from build123d import *

# Parameters (mm, degrees)
SKETCH1_W           = 21.8
SKETCH1_H           = 17.2
BOSS_EXTRUDE1_DEPTH = 1.6
SKETCH2_R           = 0.835
SKETCH2_R_2         = 1.8
CUT_EXTRUDE1_DEPTH  = 1.6


with BuildPart() as part:
    # Sketch1 → Boss-Extrude1 (new body)
    with BuildSketch(Plane.XY):
        Rectangle(SKETCH1_W, SKETCH1_H)
    extrude(amount=BOSS_EXTRUDE1_DEPTH)

    # Sketch2 → Cut-Extrude1 (cut)
    with BuildSketch(Plane.XY.offset(1.6)):
        with Locations((8.89, -7.2)):
            Circle(SKETCH2_R)
        with Locations((6.35, -7.2)):
            Circle(SKETCH2_R)
        with Locations((3.81, -7.2)):
            Circle(SKETCH2_R)
        with Locations((1.27, -7.2)):
            Circle(SKETCH2_R)
        with Locations((-1.27, -7.2)):
            Circle(SKETCH2_R)
        with Locations((-3.81, -7.2)):
            Circle(SKETCH2_R)
        with Locations((-6.35, -7.2)):
            Circle(SKETCH2_R)
        with Locations((-8.89, -7.2)):
            Circle(SKETCH2_R)
        with Locations((-8.3, 6)):
            Circle(SKETCH2_R_2)
    extrude(amount=-CUT_EXTRUDE1_DEPTH, mode=Mode.SUBTRACT)


solid = part.part
Can you work these out from the model? Positions are in its coordinate system, mm. Give positions to 0.01 mm unless a question says otherwise; leave off trailing zeros. Write each loop counter-clockwise with the first axis right and the second up, starting at its lowest first coordinate (ties: lowest second). Pieces come first, ordered by that corner, then holes. Notation, with made-up numbers: M 48.25,13 L 70.25,13 A12 ccw 70.25,33 Z; hole C -17.75,-16 d7. An arc over 180 degrees is marked long. Answer in a Markdown table with one row per item. Add a question column.
Item 1: Please list where these lines run through material, in increasing order: L1, parallel to Y at x = -8.5, z = 1.15; L2, parallel to Y at x = -8.3, z = 0.85; L3, parallel to Y at x = -1.27, z = 1 (3 decimals).
Item 2: Imagine slicing it at D-D, the plane x = -8.89. Write out the boundary of the cut face in (y, z) (3 decimals).
Item 3: Imagine slicing it at B-B, the plane y = 6. Write out the boundary of the cut face in (x, z).
Item 4: Imagine slicing it at C-C, the plane z = 0.3. State how many separate pieces and enclosed holes the cut face has, plus the area to 3 significant figures.
Item 5: For pin 1 Ø1 at (x, y) = (-8.89, -7.2) entering from +Z, with a flat end and sliding along its axis, tell me the tip position at first contact or that it passes through.
Item 6: We'd pull the mould along Y, two halves only. Please class faces 1 (the flat face through (0, 0, 0)), 2 (the cylindrical face through (4.259, -6.496, 0.811)), 3 (the flat face through (0, -8.6, 1)): released by +Y, released by -Y, zero draft, split by the parting line, or undercut.
Item 7: Imagine slicing it at A-A, the plane x = 8.89. Write out the boundary of the cut face in (y, z) (3 decimals), plus the area to 3 significant figures.
Evaluation:
| question | item | result |
|---|---|---|
| 1 | L1 | y = -8.6 to -7.94, -6.46 to 4.21, 7.79 to 8.6 |
| 1 | L2 | y = -8.6 to -7.79, -6.61 to 4.2, 7.8 to 8.6 |
| 1 | L3 | y = -8.6 to -8.035, -6.365 to 8.6 |
| 2 | outline | M -8.6,0 L -8.035,0 L -8.035,1.6 L -8.6,1.6 Z; M -6.365,0 L 4.299,0 L 4.299,1.6 L -6.365,1.6 Z; M 7.701,0 L 8.6,0 L 8.6,1.6 L 7.701,1.6 Z |
| 3 | outline | M -10.9,0 L -10.1,0 L -10.1,1.6 L -10.9,1.6 Z; M -6.5,0 L 10.9,0 L 10.9,1.6 L -6.5,1.6 Z |
| 4 | separate pieces | 1 |
| 4 | enclosed holes | 9 |
| 4 | area | 347 mm² |
| 5 | pin 1 | passes through |
| 6 | face 1 | zero draft |
| 6 | face 2 | undercut |
| 6 | face 3 | released by -Y |
| 7 | outline | M -8.6,0 L -8.035,0 L -8.035,1.6 L -8.6,1.6 Z; M -6.365,0 L 8.6,0 L 8.6,1.6 L -6.365,1.6 Z |
| 7 | area | 24.8 mm² |
